Source: CAD feature listing. Evaluate the final solid. Frame: model axes, mm. Face numbers are marked on the shaded views. A direction names the side the tool comes from. Give positions to 0.01 mm unless a question says otherwise; leave off trailing zeros. Order: outer loops, then holes, each group sorted by start corner. A loop starts at its lowest first (then second) coordinate and runs counter-clockwise, first axis right, second up. Notation, with made-up numbers: M 47.5,3.5 L 95.5,3.5 A19 cw 95.5,18.5 Z; hole C 29.5,-34.75 d2. An arc over 180 degrees is marked long. Return JSON: item names as keys, results as strings.
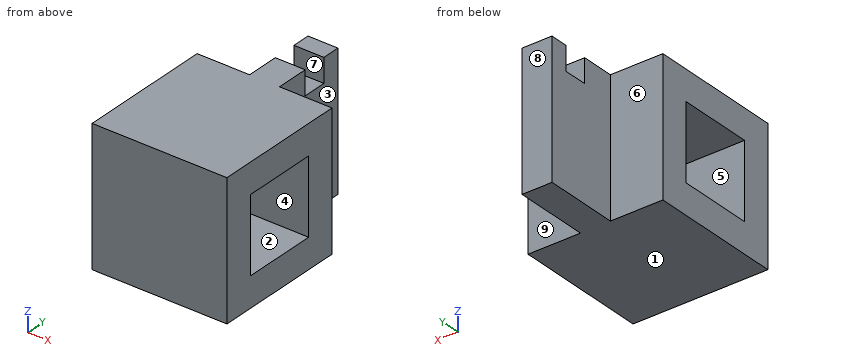
from build123d import *

# Parameters (mm, degrees)
SKETCH1_W           = 9
SKETCH1_H           = 9
SKETCH1_W_2         = 5
SKETCH1_H_2         = 5
BOSS_EXTRUDE1_DEPTH = 9
SKETCH2_W           = 2
SKETCH2_H           = 9
BOSS_EXTRUDE2_DEPTH = 5
SKETCH4_W           = 1.6
SKETCH4_H           = 1.6
CUT_EXTRUDE2_DEPTH  = 5


with BuildPart() as part:
    # Sketch1 → Boss-Extrude1 (new body)
    with BuildSketch(Plane(origin=(0, 0, 0), x_dir=(0, 0, -1), z_dir=(1, 0, 0))):
        Rectangle(SKETCH1_W, SKETCH1_H)
        Rectangle(SKETCH1_W_2, SKETCH1_H_2, mode=Mode.SUBTRACT)
    extrude(amount=BOSS_EXTRUDE1_DEPTH)

    # Sketch2 → Boss-Extrude2 (add)
    with BuildSketch(Plane(origin=(0, 4.5, 0), x_dir=(1, 0, 0), z_dir=(0, 1, 0))):
        with Locations((4.5, 0)):
            Rectangle(SKETCH2_W, SKETCH2_H)
    extrude(amount=BOSS_EXTRUDE2_DEPTH)

    # Sketch4 → Cut-Extrude2 (cut)
    with BuildSketch(Plane.ZY.offset(-3.5)):
        with Locations((3.7, 7.5)):
            Rectangle(SKETCH4_W, SKETCH4_H)
    extrude(amount=-CUT_EXTRUDE2_DEPTH, mode=Mode.SUBTRACT)


solid = part.part
1. Draft query along Z for the marked faces 1, 2, 3 and 4. Return one class per face: pulls with the +Z half, pulls with the -Z half, needs draft (parallel to the pull), parting line crosses it, or undercut.
Evaluation:
{"face 1": "pulls with the -Z half", "face 2": "undercut", "face 3": "needs draft", "face 4": "undercut"}
2. Section query B-B (y = 0). Return loops of the section in (x, z).
Evaluation:
{"outline": "M 0,-4.5 L 9,-4.5 L 9,-2.5 L 0,-2.5 Z; M 0,2.5 L 9,2.5 L 9,4.5 L 0,4.5 Z"}
3. Section query A-A (x = 2). Return loops of the section in (y, z).
Evaluation:
{"outline": "M -4.5,-4.5 L 4.5,-4.5 L 4.5,4.5 L -4.5,4.5 Z; hole M -2.5,-2.5 L 2.5,-2.5 L 2.5,2.5 L -2.5,2.5 Z"}
4. Set-up query: the marked faces 5, 6, 7, 8 and 9. Return all of +Z, -Z, +X, -X, +Y, -Y with unobstructed straight access to the full face (end or side cutting, diameter ignored); none if empty.
Evaluation:
{"face 5": "+X, -X", "face 6": "+Z, -Z, -X, +Y", "face 7": "+Z, +X, -X", "face 8": "+Z, -Z, +X, -X, +Y", "face 9": "+Z, -Z, +X, +Y"}
5. Section query C-C (z = 0.25). Return loops of the section in (x, y).
Evaluation:
{"outline": "M 0,-4.5 L 9,-4.5 L 9,-2.5 L 0,-2.5 Z; M 0,2.5 L 9,2.5 L 9,4.5 L 5.5,4.5 L 5.5,9.5 L 3.5,9.5 L 3.5,4.5 L 0,4.5 Z"}
6. Section query D-D (z = -3.25). Return loops of the section in (x, y), then the cut area to 3 significant figures.
Evaluation:
{"outline": "M 0,-4.5 L 9,-4.5 L 9,4.5 L 5.5,4.5 L 5.5,9.5 L 3.5,9.5 L 3.5,4.5 L 0,4.5 Z", "area": "91.0 mm^2"}
7. First-contact query: pin 1 (5 mm diameter, centred on y = 7.5, z = -3.5, fed in from +X); pin 2 (4 mm diameter, centred on y = 7, z = 1.5, fed in from -X); pin 3 (1.8 mm diameter, centred on x = 2, z = 2, fed in from +Y). Flat tips, straight axial feed; report the tip coordinate or a pass-through.
Evaluation:
{"pin 1": "stops at x = 5.5", "pin 2": "stops at x = 3.5", "pin 3": "stops at y = 4.5"}
8. Ray query, probe 1 along Y at (x, z) = (8, -1.75); probe 2 along Y at (x, z) = (4.5, -0.5). Return the intervals inside material, ascending.
Evaluation:
{"probe 1": "y = -4.5 to -2.5, 2.5 to 4.5", "probe 2": "y = -4.5 to -2.5, 2.5 to 9.5"}
